Build history of the part. All positions in model axes, mm. A direction names the side the tool comes from. Round coordinates to 2 decimals unless told otherwise and drop trailing zeros. Order: outer loops, then holes, each group sorted by start corner. A loop starts at its lowest first (then second) coordinate and runs counter-clockwise, first axis right, second up. Notation, with made-up numbers: (45, -25.75) - (51, -25.75) arc R30 ccw to (51, -0.75) - close; hole circle Ø2 at (-28, 18). An arc over 180 degrees is marked (long way). One line per question, with ' | ' between items. Start each with the question number.
from build123d import *

# Parameters (mm, degrees)
BOSS_EXTRUDE1_DEPTH   = 5
BOSS_EXTRUDE1_2_DEPTH = 5
BOSS_EXTRUDE2_DEPTH   = 3
FILLET1_R             = 20
FILLET2_R             = 20
CUT_EXTRUDE2_DEPTH    = 1
FILLET3_R             = 3
FILLET4_R             = 1


with BuildPart() as part:
    # Sketch1 → Boss-Extrude1 (new, symmetric)
    with BuildSketch(Plane.XY):
        with BuildLine():
            Line((-89.037246537, 5.145771556), (-69.911151418, 10.99320565))
            ThreePointArc((-69.911151418, 10.99320565), (-59.841193921, 1.000753662), (-62.6018588, -12.914413249))
            Line((-62.6018588, -12.914413249), (-81.727953919, -18.761847343))
            add(Edge.make_bspline(
                [(-81.727953919, -18.761847343), (-58.860884109, -43.388050907), (-41.130092768, -15.622946309), (-39.447011057, -12.987365142), (-38.405002213, -10)],
                knots=[2.042658164, 2.042658164, 2.042658164, 3.822478708, 3.822478708, 4.076668665, 4.076668665, 4.076668665], degree=2, weights=[1, 0.629481749, 1, 0.947083419, 0.909281691]))
            add(Edge.make_bspline(
                [(-38.405002213, -10), (-34.916949048, 0), (-38.94800166, 10)],
                knots=[4.076668665, 4.076668665, 4.076668665, 4.797306531, 4.797306531, 4.797306531], degree=2, weights=[0.909281691, 0.802112405, 0.816427746]))
            add(Edge.make_bspline(
                [(-38.94800166, 10), (-43.286972227, 20.763864888), (-53.624843095, 25.245540515), (-83.850384762, 38.348922741), (-89.037246537, 5.145771556)],
                knots=[4.797306531, 4.797306531, 4.797306531, 5.602299252, 5.602299252, 7.382119797, 7.382119797, 7.382119797], degree=2, weights=[0.816427746, 0.832418782, 1, 0.629481749, 1]))
        make_face()
    extrude(amount=BOSS_EXTRUDE1_DEPTH, both=True)



with BuildPart() as body_2:
    # Sketch1 → Boss-Extrude1 2 (new, symmetric)
    with BuildSketch(Plane.XY):
        with BuildLine():
            ThreePointArc((193.385488342, 0), (182.162671381, 15.633340627), (163.761083594, 10))
            ThreePointArc((163.761083594, 10), (160.385488342, 0), (163.761083594, -10))
            ThreePointArc((163.761083594, -10), (182.162671381, -15.633340627), (193.385488342, 0))
        make_face()
        Polygon((170.635488342, 10.825317547), (173.984853248, 10.825317547), (176.885488342, 12.5), (179.786123437, 10.825317547), (183.135488342, 10.825317547), (184.810170795, 7.924682453), (187.71080589, 6.25), (187.71080589, 2.900635095), (189.385488342, 0), (187.71080589, -2.900635095), (187.71080589, -6.25), (184.810170795, -7.924682453), (183.135488342, -10.825317547), (179.786123437, -10.825317547), (176.885488342, -12.5), (173.984853248, -10.825317547), (170.635488342, -10.825317547), (168.96080589, -7.924682453), (166.060170795, -6.25), (166.060170795, -2.900635095), (164.385488342, 0), (166.060170795, 2.900635095), (166.060170795, 6.25), (168.96080589, 7.924682453), align=None, mode=Mode.SUBTRACT)
    extrude(amount=BOSS_EXTRUDE1_2_DEPTH, both=True)


with BuildPart() as part_1:
    add(part.part)

    add(body_2.part)  # Boss-Extrude2 merges body 2
    # Sketch1<4> → Boss-Extrude2 (add, symmetric)
    with BuildSketch(Plane.XY):
        with BuildLine():
            Line((163.761083594, 10), (-38.94800166, 10))
            add(Edge.make_bspline(
                [(-38.405002213, -10), (-34.916949048, 0), (-38.94800166, 10)],
                knots=[4.076668665, 4.076668665, 4.076668665, 4.797306531, 4.797306531, 4.797306531], degree=2, weights=[0.909281691, 0.802112405, 0.816427746]))
            Line((-38.405002213, -10), (163.761083594, -10))
            ThreePointArc((163.761083594, -10), (160.385488342, 0), (163.761083594, 10))
        make_face()
    extrude(amount=BOSS_EXTRUDE2_DEPTH, both=True)

    # Fillet1
    # the kernel refuses this fillet: 20 mm, written as the material it adds along each edge
    with BuildSketch(Plane(origin=(-38.94800166, 10, 0), x_dir=(-0.507799469280601, 0.8614753037657783, 0), z_dir=(0, 0, -1))) as fillet1_piece_1:
        with BuildLine():
            CenterArc((11.560223387, 19.773854944), FILLET1_R, 210.517364345, 50.858287997)
            Line((-5.669282689, 9.617865559), (-6.01387281, 9.414745771))
            Line((-6.01387281, 9.414745771), (-0.344590122, -0.203119788))
            Line((-0.344590122, -0.203119788), (0.059556935, -0.395541365))
            ThreePointArc((0.059556935, -0.395541365), (4.280578149, -0.078560147), (8.501131211, -0.395477099))
            Line((8.501131211, -0.395477099), (8.561113411, 0))
        make_face()
    fillet1_piece_1_solid = extrude(amount=3, mode=Mode.PRIVATE)
    with BuildSketch(Plane(origin=(-38.405002213, -10, 0), x_dir=(-0.4780913374533499, -0.8783101235053977, 0), z_dir=(0, 0, 1))) as fillet1_piece_2:
        with BuildLine():
            CenterArc((12.033263145, 19.726488271), FILLET1_R, 208.560818285, 51.952664674)
            Line((-5.532939325, 10.164661522), (-5.884263374, 9.973424987))
            Line((-5.884263374, 9.973424987), (-0.351324049, -0.191236535))
            Line((-0.351324049, -0.191236535), (0.064860434, -0.394706377))
            ThreePointArc((0.064860434, -0.394706377), (4.368504422, -0.040514317), (8.671026811, -0.394529765))
            Line((8.671026811, -0.394529765), (8.736953014, 0))
        make_face()
    fillet1_piece_2_solid = extrude(amount=3, mode=Mode.PRIVATE)
    with BuildSketch(Plane(origin=(-38.405002213, -10, 0), x_dir=(-0.4780913374533499, -0.8783101235053977, 0), z_dir=(0, 0, -1))) as fillet1_piece_3:
        with BuildLine():
            CenterArc((12.033263145, -19.726488271), FILLET1_R, 99.486517041, 51.952664674)
            Line((-5.532939325, -10.164661522), (-5.884263374, -9.973424987))
            Line((-5.884263374, -9.973424987), (-0.351324049, 0.191236535))
            Line((-0.351324049, 0.191236535), (0.064860434, 0.394706377))
            ThreePointArc((0.064860434, 0.394706377), (4.368504422, 0.040514317), (8.671026811, 0.394529765))
            Line((8.671026811, 0.394529765), (8.736953014, 0))
        make_face()
    fillet1_piece_3_solid = extrude(amount=3, mode=Mode.PRIVATE)
    with BuildSketch(Plane(origin=(-38.94800166, 10, 0), x_dir=(-0.507799469280601, 0.8614753037657783, 0), z_dir=(0, 0, 1))) as fillet1_piece_4:
        with BuildLine():
            CenterArc((11.560223387, -19.773854944), FILLET1_R, 98.624347659, 50.858287997)
            Line((-5.669282689, -9.617865559), (-6.01387281, -9.414745771))
            Line((-6.01387281, -9.414745771), (-0.344590122, 0.203119788))
            Line((-0.344590122, 0.203119788), (0.059556935, 0.395541365))
            ThreePointArc((0.059556935, 0.395541365), (4.280578149, 0.078560147), (8.501131211, 0.395477099))
            Line((8.501131211, 0.395477099), (8.561113411, 0))
        make_face()
    fillet1_piece_4_solid = extrude(amount=3, mode=Mode.PRIVATE)
    add([fillet1_piece_1_solid, fillet1_piece_2_solid, fillet1_piece_3_solid, fillet1_piece_4_solid])

    # Fillet2
    # the kernel refuses this fillet: 20 mm, written as the material it adds along each edge
    with BuildSketch(Plane(origin=(163.761083594, -10, 0), x_dir=(0.7228612548390331, -0.6909932027542227, 0), z_dir=(0, 0, -1))) as fillet2_piece_1:
        with BuildLine():
            CenterArc((8.278251992, 19.754529721), FILLET2_R, 226.291219019, 34.722762927)
            Line((-5.541612063, 5.297304624), (0, 0))
            ThreePointArc((0, 0), (2.577191658, 0.20251298), (5.154383316, 0))
        make_face()
    extrude(amount=3)
    with BuildSketch(Plane(origin=(163.761083594, 10, 0), x_dir=(-1, 0, 0), z_dir=(0, 0, -1)), Plane(origin=(163.761083594, -10, 0), x_dir=(-1, 0, 0), z_dir=(0, 0, 1))) as fillet2_piece_2:
        with BuildLine():
            CenterArc((7.666218138, 20), FILLET2_R, 235.277237073, 34.722762927)
            ThreePointArc((-3.725903992, 3.561643836), (-1.723016903, 1.927210705), (0, 0))
            Line((0, 0), (7.666218138, 0))
        make_face()
    extrude(amount=3)
    with BuildSketch(Plane(origin=(163.761083594, 10, 0), x_dir=(-1, 0, 0), z_dir=(0, 0, 1))) as fillet2_piece_3:
        with BuildLine():
            CenterArc((7.666218138, -20), FILLET2_R, 90, 34.722762927)
            ThreePointArc((-3.725903992, -3.561643836), (-1.723016903, -1.927210705), (0, 0))
            Line((0, 0), (7.666218138, 0))
        make_face()
    extrude(amount=3)

    # Sketch4 → Cut-Extrude2 (cut)
    with BuildSketch(Plane.XY.offset(3)):
        with BuildLine():
            Line((156.094865456, 6.5), (-27.783589266, 6.5))
            ThreePointArc((-27.783589266, 6.5), (-24.615419845, 0.197075053), (-26.832026734, -6.5))
            Line((-26.832026734, -6.5), (156.094865456, -6.5))
            ThreePointArc((156.094865456, -6.5), (153.402477301, 0), (156.094865456, 6.5))
        make_face()
    extrude(amount=-CUT_EXTRUDE2_DEPTH, mode=Mode.SUBTRACT)

    # Fillet3
    fillet3_edges = [part_1.edges().sort_by_distance(p)[0] for p in [
        (-27.783589266, 6.5, 2.5),
        (156.094865456, 6.5, 2.5),
        (156.094865456, -6.5, 2.5),
        (-26.832026734, -6.5, 2.5),
    ]]
    fillet(fillet3_edges, radius=FILLET3_R)

    # Fillet4
    fillet4_edges = [part_1.edges().sort_by_distance(p)[0] for p in [
        (-36.865276066, 0.047607181, 5),
        (182.162671381, 15.633340627, 5),
    ]]
    fillet(fillet4_edges, radius=FILLET4_R)


solid = part_1.part
Item 1: Slice it at B-B (x = -33). Write the cut outline in (y, z).
Item 2: Pull direction Y, two halves, no side cores. Call faces 4 (the face through (185, -8, 5)), 5 (the face through (161.982, 10.886, -0.042)), 6 (the face through (-79.61, 8.03, 0.07)): released by +Y, released by -Y, zero draft, split by the parting line, or undercut.
Item 3: Pin check, flat tips, straight feed: pin 1 (4 mm diameter, centred on x = 128, y = 8.5, fed in from -Z); pin 2 (2.5 mm diameter, centred on y = -4, z = -1.5, fed in from -X); pin 3 (3.5 mm diameter, centred on y = -5, z = -3.5, fed in from +X); pin 4 (1 mm diameter, centred on y = 5, z = -2, fed in from -X). Stop position of each tip, or through.
Item 4: 3-axis set-ups, long thin cutter, end or side, ignore diameter. For faces 1 (the face through (63, 0, 2)), 2 (the face through (65, 10, 0)), 3 (the face through (-59.903, 1.198, 0.07)): which of +Z, -Z, +X, -X, +Y, -Y reach the whole face in a straight line?
Item 5: Wall check: line 1 along Y through (x, z) = (141.5, 2.5); line 2 along X through (y, z) = (-1, 2.25); line 3 along X through (y, z) = (2, 4). Give the ranges that are in metal, low to high. Write a range as [from, to].
Item 6: Slice it at A-A (x = 117). Write the cut outline in (y, z), plus the area to 3 significant figures.
A:
1) outline: (-10.97, -3) - (10.69, -3) - (10.69, 3) - (-10.97, 3) - close
2) face 4: zero draft | face 5: released by +Y | face 6: undercut
3) pin 1: z = -3 | pin 2: x = -59.3 | pin 3: x = 193.06 | pin 4: x = -89.04
4) face 1: +Z | face 2: +Z, -Z, +Y | face 3: +Z, -Z
5) line 1: [-10, -6.5], [6.5, 10] | line 2: [-59.38, -24.61], [153.46, 164.96], [188.81, 193.36] | line 3: [-60.19, -36.99], [160.51, 165.54], [188.23, 193.26]
6) outline: (-10, -3) - (10, -3) - (10, 3) - (6.5, 3) - (6.5, 2) - (-6.5, 2) - (-6.5, 3) - (-10, 3) - close | area: 107 mm^2
